Model file for the job. Use its own axes, mm. Round coordinates to 2 decimals unless told otherwise and drop trailing zeros. Loops run counter-clockwise (first coordinate to the right, second up) from the corner with the lowest first, then second, coordinate; pieces in that order, holes last. Notation, with made-up numbers: M -3,6 L 39,6 A21 ccw 39,16 Z; hole C -9,-5 d9. An arc over 180 degrees is marked long. Answer in a Markdown table with one row per item.
from build123d import *

# Parameters (mm, degrees)
SCHIZZO1_W                   = 50
SCHIZZO1_H                   = 2
ESTRUSIONE_ESTRUSIONE1_DEPTH = 5
SCHIZZO2_W                   = 50
SCHIZZO2_H                   = 1
ESTRUSIONE_ESTRUSIONE2_DEPTH = 40
SCHIZZO3_W                   = 45
SCHIZZO3_H                   = 1
ESTRUSIONE_ESTRUSIONE3_DEPTH = 0.5


with BuildPart() as part:
    # Schizzo1 → Estrusione-Estrusione1 (new body)
    with BuildSketch(Plane.XY):
        with Locations((15.607042649, 0.147727273)):
            Rectangle(SCHIZZO1_W, SCHIZZO1_H)
    extrude(amount=ESTRUSIONE_ESTRUSIONE1_DEPTH)

    # Schizzo2 → Estrusione-Estrusione2 (add)
    with BuildSketch(Plane.XY.offset(5)):
        with Locations((15.607042649, 0.147727273)):
            Rectangle(SCHIZZO2_W, SCHIZZO2_H)
    extrude(amount=ESTRUSIONE_ESTRUSIONE2_DEPTH)

    # Schizzo3 → Estrusione-Estrusione3 (add)
    with BuildSketch(Plane.XZ.offset(0.352272727)):
        with Locations((15.607042649, 44.5)):
            Rectangle(SCHIZZO3_W, SCHIZZO3_H)
        with Locations((15.607042649, 42)):
            Rectangle(SCHIZZO3_W, SCHIZZO3_H)
        with Locations((15.607042649, 39.5)):
            Rectangle(SCHIZZO3_W, SCHIZZO3_H)
        with Locations((15.607042649, 37)):
            Rectangle(SCHIZZO3_W, SCHIZZO3_H)
        with Locations((15.607042649, 34.5)):
            Rectangle(SCHIZZO3_W, SCHIZZO3_H)
        with Locations((15.607042649, 32)):
            Rectangle(SCHIZZO3_W, SCHIZZO3_H)
        with Locations((15.607042649, 29.5)):
            Rectangle(SCHIZZO3_W, SCHIZZO3_H)
        with Locations((15.607042649, 27)):
            Rectangle(SCHIZZO3_W, SCHIZZO3_H)
        with Locations((15.607042649, 24.5)):
            Rectangle(SCHIZZO3_W, SCHIZZO3_H)
        with Locations((15.607042649, 22)):
            Rectangle(SCHIZZO3_W, SCHIZZO3_H)
        with Locations((15.607042649, 19.5)):
            Rectangle(SCHIZZO3_W, SCHIZZO3_H)
        with Locations((15.607042649, 17)):
            Rectangle(SCHIZZO3_W, SCHIZZO3_H)
    extrude(amount=ESTRUSIONE_ESTRUSIONE3_DEPTH)


solid = part.part
1. Mould opens along Z. For faces 1 (the flat face through (15, 0, 0)), 2 (the flat face through (15, 0, 45)), 3 (the flat face through (15.3, -0.352, 20.3)), 4 (the flat face through (15, 0.648, 25)) say: +Z half, -Z half, draft (parallel to the pull), parting line (faces both ways), or undercut.
Verdict:
| item | result |
|---|---|
| face 1 | -Z half |
| face 2 | +Z half |
| face 3 | undercut |
| face 4 | draft |
2. Pin check, flat tip, straight feed: pin 1 (1.5 mm diameter, centred on x = 5.5, z = 8.5, fed in from +Y). Stop position of the tip, or through.
Verdict:
| item | result |
|---|---|
| pin 1 | stops at y = 0.65 |
3. Wall check: probe 1 along Y at (x, z) = (6, 31); probe 2 along Z at (x, y) = (25, 1); probe 3 along Y at (x, z) = (9.5, 24.5). Give the ranges that are in metal, low to high.
Verdict:
| item | result |
|---|---|
| probe 1 | y = -0.35 to 0.65 |
| probe 2 | z = 0 to 5 |
| probe 3 | y = -0.85 to 0.65 |
4. Saw through at A-A (z = 8.5). Write the cut outline in (x, y).
Verdict:
| item | result |
|---|---|
| outline | M -9.39,-0.35 L 40.61,-0.35 L 40.61,0.65 L -9.39,0.65 Z |
